Can you work these out from the model? Positions are in its coordinate system, mm. A direction names the side the tool comes from. Round coordinates to 2 decimals unless told otherwise and drop trailing zeros. Loops run counter-clockwise (first coordinate to the right, second up) from the corner with the lowest first, then second, coordinate; pieces in that order, holes last. Notation, with made-up numbers: (85.5, 69.5) - (125.5, 69.5) arc R12 cw to (125.5, 90.5) - close; hole circle Ø2 at (63, -35.75). An arc over 180 degrees is marked (long way). Answer as CSV lines item,"result".
```python
from build123d import *

# Parameters (mm, degrees)
SKETCH001_W  = 3.8
SKETCH001_H  = 0.7
POCKET_DEPTH = 0.6


with BuildPart() as part:
    # Sketch → Revolution (revolve)
    with BuildSketch(Plane.YZ):
        with BuildLine():
            Line((0, 1.603002), (0, 0))
            Line((0, 0), (21.3, 0))
            Line((21.3, 0), (21.3, 0.755))
            Line((21.3, 0.755), (21.158549, 1))
            Line((21.158549, 1), (1.3, 1))
            Line((1.3, 1), (1.3, 1.9))
            Line((1.3, 1.9), (0.182569, 1.802237))
            ThreePointArc((0.182569, 1.802237), (0.052546, 1.738118), (0, 1.603002))
        make_face()
    revolve(axis=Axis((0, 0, 0), (0, 1, 0)))

    # Sketch001 → Pocket (cut)
    with BuildSketch(Plane(origin=(0, 0, 0), x_dir=(0, 0, -1), z_dir=(0, -1, 0))):
        Rectangle(SKETCH001_W, SKETCH001_H)
    extrude(amount=-POCKET_DEPTH, mode=Mode.SUBTRACT)


solid = part.part
```
Q1. I'm going to push flat-ended pins straight in: pin 1 Ø2 at (y, z) = (17.5, 0) entering from +X; pin 2 Ø1 at (y, z) = (3, -1) entering from -X; pin 3 Ø1 at (x, y) = (0.5, 17) entering from -Z. Where does each tip first touch, or does it pass through?
Checks:
pin 1,"x = 1"
pin 2,"x = -0.87"
pin 3,"z = -1"
Q2. Imagine slicing it at B-B (x = 0). Write out the boundary of the cut face in (y, z) (3 decimals).
Checks:
outline,"(0.6, -1.839) - (1.3, -1.9) - (1.3, -1) - (21.159, -1) - (21.3, -0.755) - (21.3, 0.755) - (21.159, 1) - (1.3, 1) - (1.3, 1.9) - (0.6, 1.839) - close"
Q3. Imagine slicing it at A-A (z = 0). Write out the boundary of the cut face in (x, y) (3 decimals).
Checks:
outline,"(-1.9, 1.3) - (-1.802, 0.183) arc R0.2 ccw to (-1.603, 0) - (-0.35, 0) - (-0.35, 0.6) - (0.35, 0.6) - (0.35, 0) - (1.603, 0) arc R0.2 ccw to (1.802, 0.183) - (1.9, 1.3) - (1, 1.3) - (1, 21.159) - (0.755, 21.3) - (-0.755, 21.3) - (-1, 21.159) - (-1, 1.3) - close"
Q4. On a 3-axis mill with a long thin cutter (end or side, diameter ignored), from which of +Z, -Z, +X, -X, +Y, -Y can I reach the whole of each face in a straight line? I mean faces 1 (the flat face through (0, 21.3, 0)), 2 (the cylindrical face through (-1, 11, 0)). Say none if no direction works.
Checks:
face 1,"+Z, -Z, +X, -X, +Y"
face 2,"+Y"
Q5. If I drill on line 1 along Y through (x, z) = (-1.3, 0.45); line 2 along X through (y, z) = (1.5, -0.1); line 3 along Y through (x, z) = (0.15, -0.7), over which ranges is the centre line in solid material (lowest first)? Write a range as [from, to].
Checks:
line 1,"[0, 1.3]"
line 2,"[-0.99, 0.99]"
line 3,"[0.6, 21.3]"
Q6. Imagine slicing it at C-C (y = 9.25). Write out the boundary of the cut face in (x, z), then the cut area to 3 significant figures.
Checks:
outline,"circle Ø2 at (0, 0)"
area,"3.14 mm²"
